from build123d import *

# Parameters (mm, degrees)
F0_W          = 130.5
F0_H          = 2
F1_DEPTH      = 3
F0_W_2        = 142.5
F0_H_2        = 78
F0_W_3        = 7
F2_DEPTH      = 3
F2_DEPTH_BACK = 12.7
F3_W          = 5.5
F3_H          = 7.5
F4_DEPTH      = 12.7
F6_DEPTH      = 4.001
F8_DEPTH      = 4.001
F9_DEPTH      = 0.4
F10_DEPTH     = 2
F11_DEPTH     = 2


with BuildPart() as f1:
    # F0 (on Front) → F1 (new body)
    with BuildSketch(Plane.XZ):
        Polygon((67.25, 35), (65.25, 35), (65.25, 33), (65.25, -33), (65.25, -35), (67.25, -35), align=None)
        with Locations((0, 34)):
            Rectangle(F0_W, F0_H)
        Polygon((-65.25, 35), (-67.25, 35), (-67.25, -35), (-65.25, -35), (-65.25, -33), (-65.25, 33), align=None)
        with Locations((0, -34)):
            Rectangle(F0_W, F0_H)
    extrude(amount=-F1_DEPTH)

    # F0 (on Front) → F2 (join, two sides)
    with BuildSketch(Plane.XZ) as f2_sk:
        Rectangle(F0_W_2, F0_H_2)
        Polygon((-67.25, -35), (-67.25, 35), (-65.25, 35), (65.25, 35), (67.25, 35), (67.25, -35), (65.25, -35), (-65.25, -35), align=None, mode=Mode.SUBTRACT)
        with Locations((-74.75, 0)):
            Rectangle(F0_W_3, F0_H_2)
        with Locations((74.75, 0)):
            Rectangle(F0_W_3, F0_H_2)
    extrude(amount=-F2_DEPTH)
    extrude(f2_sk.sketch, amount=F2_DEPTH_BACK)

    # F3 (on face) → F4 (cut)
    with BuildSketch(Plane.XZ.offset(12.7)):
        with Locations((-75.5, 3.75)):
            Rectangle(F3_W, F3_H)
        with Locations((-70, 3.75)):
            Rectangle(F3_W, F3_H)
        with Locations((-70, -3.75)):
            Rectangle(F3_W, F3_H)
        with Locations((-75.5, -3.75)):
            Rectangle(F3_W, F3_H)
    extrude(amount=-F4_DEPTH, mode=Mode.SUBTRACT)

    # F5 (on face) → F6 (cut, through all)
    with BuildSketch(Plane(origin=(0, 0, 35), x_dir=(1, 0, 0), z_dir=(0, 0, -1))):
        Polygon((47.75, 3.35), (47.75, 6.35), (47.75, 9.35), (32.75, 9.35), (32.75, 3.35), align=None)
    extrude(amount=-F6_DEPTH, mode=Mode.SUBTRACT)

    # F7 (on face) → F8 (cut, through all)
    with BuildSketch(Plane.XY.offset(-35)):
        Polygon((37.25, -9.35), (37.25, -6.35), (37.25, -3.35), (11.25, -3.35), (11.25, -9.35), align=None)
    extrude(amount=-F8_DEPTH, mode=Mode.SUBTRACT)

    # F9 (add): faces of the model
    f9_faces = [f1.faces().sort_by_distance(p)[0] for p in [
        (67.25, -6.35, 0),
        (65.25, 1.5, 0),
    ]]
    extrude(f9_faces, amount=F9_DEPTH)

    # F10 (cut): a face of the model
    f10_faces = [f1.faces().sort_by_distance(p)[0] for p in [
        (24.25, -3.35, -37),
    ]]
    extrude(f10_faces, amount=-F10_DEPTH, mode=Mode.SUBTRACT)

    # F11 (cut): a face of the model
    f11_faces = [f1.faces().sort_by_distance(p)[0] for p in [
        (40.25, -3.35, 37),
    ]]
    extrude(f11_faces, amount=-F11_DEPTH, mode=Mode.SUBTRACT)


solid = f1.part
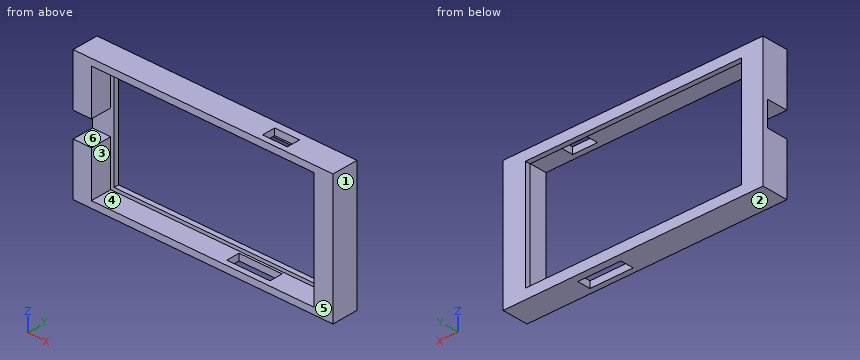
Can you work these out from the model? Positions are in its coordinate system, mm. Face numbers are marked on the shaded views. A direction names the side the tool comes from. Give positions to 0.01 mm unless a question says otherwise; leave off trailing zeros. Write each loop counter-clockwise with the first axis right and the second up, starting at its lowest first coordinate (ties: lowest second). Pieces come first, ordered by that corner, then holes. Notation, with made-up numbers: (21, -1.5) -> (57, -1.5) arc R15 cw to (57, 17.5) -> close; hole circle Ø5 at (-37.75, -25.5). An arc over 180 degrees is marked (long way). Answer as a JSON object with one key per item and string values. Group by question number.
Item 1: Suppose I cut it at B-B (x = -27). Please give me the cut outline in (y, z), plus the area to 3 significant figures.
Item 2: Suppose I cut it at C-C (x = 18.5). Please give me the cut outline in (y, z), plus the area to 3 significant figures.
Item 3: We'd pull the mould along Z, two halves only. Please class the marked faces 1, 2 and 3: +Z half, -Z half, draft (parallel to the pull), parting line (faces both ways), or undercut.
Item 4: For the marked faces 4, 5 and 6, which set-ups out of +Z, -Z, +X, -X, +Y, -Y let a thin tool reach every point of the face, with its end or its side?
Item 5: Suppose I cut it at A-A (z = 2). Please give me the cut outline in (x, y).
Item 6: Suppose I cut it at D-D (z = -20). Please give me the cut outline in (x, y).
Item 7: I'm going to push a flat-ended pin straight in: P1, Ø3, axis at y = -9.5, z = 0.5, coming from the -X side. Where does the tip first touch, or does it pass through?
Item 8: Please list where these lines run through material, in increasing order: line 1 (X direction, y = -10, z = -23); line 2 (Z direction, x = 6, y = -8.75); line 3 (Z direction, x = -35, y = 1.5). Write a range as [from, to].
Findings:
{
 "1": {"outline": "(-12.7, -39) -> (3, -39) -> (3, -33) -> (0, -33) -> (0, -35) -> (-12.7, -35) -> close; (-12.7, 35) -> (0, 35) -> (0, 33) -> (3, 33) -> (3, 39) -> (-12.7, 39) -> close", "area": "138 mm²"},
 "2": {"outline": "(-12.7, -39) -> (-9.35, -39) -> (-9.35, -35) -> (-12.7, -35) -> close; (-12.7, 35) -> (0, 35) -> (0, 33) -> (3, 33) -> (3, 39) -> (-12.7, 39) -> close; (-1.35, -39) -> (3, -39) -> (3, -33) -> (0, -33) -> (0, -35) -> (-1.35, -35) -> close", "area": "106 mm²"},
 "3": {"face 1": "draft", "face 2": "-Z half", "face 3": "undercut"},
 "4": {"face 4": "-Y", "face 5": "+Z, -Z, +X, -X, -Y", "face 6": "-X, -Y"},
 "5": {"outline": "(-78.25, 0) -> (-65.25, 0) -> (-65.25, 3) -> (-78.25, 3) -> close; (64.85, 0) -> (66.85, 0) -> (66.85, -12.7) -> (78.25, -12.7) -> (78.25, 3) -> (64.85, 3) -> close"},
 "6": {"outline": "(-78.25, -12.7) -> (-67.25, -12.7) -> (-67.25, 0) -> (-65.25, 0) -> (-65.25, 3) -> (-78.25, 3) -> close; (64.85, 0) -> (66.85, 0) -> (66.85, -12.7) -> (78.25, -12.7) -> (78.25, 3) -> (64.85, 3) -> close"},
 "7": {"P1": "stops at x = 66.85"},
 "8": {"line 1": "x = [-78.25, -67.25], [66.85, 78.25]", "line 2": "z = [-39, -35], [35, 39]", "line 3": "z = [-39, -33], [33, 39]"}
}
